Design review of the part built by this model. Coordinates are the model's own, in mm. A direction names the side the tool comes from. Give positions to 0.01 mm unless a question says otherwise; leave off trailing zeros. Write each loop counter-clockwise with the first axis right and the second up, starting at its lowest first coordinate (ties: lowest second). Pieces come first, ordered by that corner, then holes. Notation, with made-up numbers: (-24, 58.5) -> (-15, 58.5) arc R13 cw to (-15, 72.5) -> close; hole circle Ø3 at (-38, 76.25). An arc over 180 degrees is marked (long way). Answer as a JSON object with one key per item and string values.
```python
from build123d import *

# Parameters (mm, degrees)
FILLET1_R   = 0.2
HEX_2_DEPTH = 1.56


with BuildPart() as part:
    # BodySke → BaseBody (revolve)
    with BuildSketch(Plane.XY):
        with BuildLine():
            Line((32.75, 0), (32.75, 2.055))
            Line((32.75, 2.055), (32.305, 2.5))
            Line((32.305, 2.5), (2.75, 2.5))
            Line((2.75, 2.5), (2.75, 4.75))
            Line((2.75, 4.75), (2.37, 4.75))
            ThreePointArc((2.37, 4.75), (0.992680215, 3.754414901), (0, 2.375))
            Line((0, 2.375), (0, 0))
            Line((0, 0), (32.75, 0))
        make_face()
    revolve(axis=Axis((0, 0, 0), (1, 0, 0)))

    # Fillet1
    fillet1_edges = [part.edges().sort_by_distance(p)[0] for p in [
        (2.75, -2.5, 0),
    ]]
    fillet(fillet1_edges, radius=FILLET1_R)

    # Sketch2 → PreBroach (revolve, cut)
    with BuildSketch(Plane.XY):
        Polygon((0, 1.5), (1.56, 1.5), (2.426025404, 0), (0, 0), align=None)
    revolve(axis=Axis((0, 0, 0), (1, 0, 0)), mode=Mode.SUBTRACT)

    # Sketch3 → Hex 2 (cut)
    with BuildSketch(Plane(origin=(0, 0, 0), x_dir=(0, 0, -1), z_dir=(1, 0, 0))):
        Polygon((-1.5, -0.866025404), (-1.5, 0.866025404), (0, 1.732050808), (1.5, 0.866025404), (1.5, -0.866025404), (0, -1.732050808), align=None)
    extrude(amount=HEX_2_DEPTH, mode=Mode.SUBTRACT)


solid = part.part
```
(1) For faces 4 (the flat face through (0.769, 1.293, 0.76)), 5 (the cylindrical face through (17.42, -0.54, -2.44)), 6 (the flat face through (32.75, 0, 0)), list the 3-axis set-ups (+Z, -Z, +X, -X, +Y, -Y) from which the entire face can be reached by the end or side of a thin tool; tool diameter is ignored.
Here are the results:
{"face 4": "-X", "face 5": "+X", "face 6": "+Z, -Z, +X, +Y, -Y"}
(2) Clearance check with flat-ended pins moving along their axes: pin 1 (0.8 mm diameter, centred on x = 1, y = 0, fed in from -Z); pin 2 (4 mm diameter, centred on x = 9, y = 3.5, fed in from +Z); pin 3 (0.8 mm diameter, centred on x = 1, y = 0, fed in from +Z). State where each tip first meets the part, or that it passes through.
Here are the results:
{"pin 1": "stops at z = -4.12", "pin 2": "stops at z = 2", "pin 3": "stops at z = 4.12"}
(3) We need section A-A, the plane x = 5. State the section outline as (y, z) points.
Here are the results:
{"outline": "circle Ø5 at (0, 0)"}
(4) For line 1 along X through (y, z) = (4, 1.75); line 2 along Y through (x, z) = (22.5, 2); line 3 along Z through (x, y) = (30, 1.5), list the stretches that pass through material, from the lowest coordinate up.
Here are the results:
{"line 1": "x = 1.72 to 2.75", "line 2": "y = -1.5 to 1.5", "line 3": "z = -2 to 2"}
(5) We need section B-B, the plane z = 4. State the section outline as (x, y) points, then the cut area to 3 significant figures.
Here are the results:
{"outline": "(2.37, -2.56) -> (2.75, -2.56) -> (2.75, 2.56) -> (2.37, 2.56) arc R3.5 ccw to start", "area": "5.90 mm²"}
(6) The part is to be moulded in two halves that separate along Z. For faces 1 (the cylindrical face through (2.557, 2.192, -4.214)), 2 (the flat face through (1, 0, 1.5)), 3 (the flat face through (2.75, -2.04, -2.04)), say which applies: +Z half, -Z half, draft (parallel to the pull), parting line (faces both ways), or undercut.
Here are the results:
{"face 1": "parting line", "face 2": "undercut", "face 3": "draft"}
